The listing builds one solid part. Answer for the finished solid, in the listing's coordinates (mm). Face numbers are marked on the shaded views. A direction names the side the tool comes from. Round coordinates to 2 decimals unless told otherwise and drop trailing zeros. Write each loop counter-clockwise with the first axis right and the second up, starting at its lowest first coordinate (ties: lowest second). Pieces come first, ordered by that corner, then holes. Notation, with made-up numbers: M 66.5,47 L 91.5,47 A15 cw 91.5,76 Z; hole C 20,43.25 d1. An arc over 180 degrees is marked long. One line per item, written item: value. Start each with the question number.
(1) For the marked faces 4, 5 and 6, determine the directions among +Z, -Z, +X, -X, +Y, -Y from which every point of the face is accessible in a straight line to the end or side of a thin tool.
(2) Section A-A (y = 2) is taken. Determine the outline of the cut face in (x, z), plus the area to 3 significant figures.
(3) Section D-D (z = 6) is taken. Determine the outline of the cut face in (x, y), plus the area to 3 significant figures.
(4) Section C-C (y = 0) is taken. Determine the outline of the cut face in (x, z), plus the area to 4 significant figures.
(5) For a pull along Y with two mould halves and no side action, classify the marked faces 1, 2 and 3 as released by +Y, released by -Y, zero draft, split by the parting line, or undercut.
(6) Given P1, Ø2, axis at y = -2.5, z = 3.5, coming from the +X side; P2, Ø3, axis at y = 2, z = 8, coming from the +X side; P3, Ø2, axis at x = -5, y = 5.5, coming from the +Z side, each flat-ended and moving along its own axis, determine where each tip first touches the part or whether it passes through.
(7) Section B-B (x = 0) is taken. Determine the outline of the cut face in (y, z).
(8) Consider probe 1 along Y at (x, z) = (0, 6.5); probe 2 along Z at (x, y) = (5.25, 4); probe 3 along X at (y, z) = (0, 7.5). Determine where each line is inside the solid, lowest interval first.
```python
from build123d import *

# Parameters (mm, degrees)
BOX_W             = 11
BOX_H             = 1.5
BOX_DEPTH         = 15
CYLINDER002_R     = 4
CYLINDER002_DEPTH = 15
CYLINDER001_R     = 8
CYLINDER001_DEPTH = 1.5
CYLINDER_R        = 5.5
CYLINDER_DEPTH    = 10


with BuildPart() as cube:
    # Box → Box (new body)
    with BuildSketch(Plane(origin=(0, -0.75, 0), x_dir=(1, 0, 0), z_dir=(0, 0, 1))):
        with Locations((5.5, 0.75)):
            Rectangle(BOX_W, BOX_H)
    extrude(amount=BOX_DEPTH)


with BuildPart() as hole:
    # Cylinder002 → Cylinder002 (new body)
    with BuildSketch(Plane.XY):
        Circle(CYLINDER002_R)
    extrude(amount=CYLINDER002_DEPTH)


with BuildPart() as base:
    # Cylinder001 → Cylinder001 (new body)
    with BuildSketch(Plane.XY):
        Circle(CYLINDER001_R)
    extrude(amount=CYLINDER001_DEPTH)


with BuildPart() as cut001:
    # Cylinder → Cylinder (new body)
    with BuildSketch(Plane.XY):
        Circle(CYLINDER_R)
    extrude(amount=CYLINDER_DEPTH)

    # Fusion: union base
    add(base.part)

    # Cut: cut hole
    add(hole.part, mode=Mode.SUBTRACT)

    # Cut001: cut Cube
    add(cube.part, mode=Mode.SUBTRACT)


solid = cut001.part
```
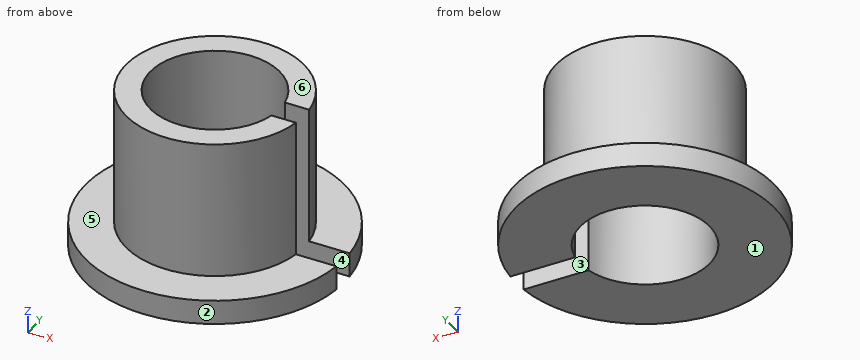
Recorded:
1. face 4: +Z, -Z, +X
1. face 5: +Z
1. face 6: +Z, +X, -X, +Y, -Y
2. outline: M -7.75,0 L -3.46,0 L -3.46,10 L -5.12,10 L -5.12,1.5 L -7.75,1.5 Z; M 3.46,0 L 7.75,0 L 7.75,1.5 L 5.12,1.5 L 5.12,10 L 3.46,10 Z
2. area: 41.1 mm2
3. outline: M 3.93,-0.75 A4 cw long 3.93,0.75 L 5.45,0.75 A5.5 ccw long 5.45,-0.75 Z
3. area: 42.5 mm2
4. outline: M -8,0 L -4,0 L -4,10 L -5.5,10 L -5.5,1.5 L -8,1.5 Z
4. area: 18.75 mm2
5. face 1: zero draft
5. face 2: split by the parting line
5. face 3: undercut
6. P1: stops at x = 5.29
6. P2: stops at x = 5.45
6. P3: stops at z = 1.5
7. outline: M -8,0 L -4,0 L -4,10 L -5.5,10 L -5.5,1.5 L -8,1.5 Z; M 4,0 L 8,0 L 8,1.5 L 5.5,1.5 L 5.5,10 L 4,10 Z
8. probe 1: y = -5.5 to -4, 4 to 5.5
8. probe 2: z = 0 to 1.5
8. probe 3: x = -5.5 to -4
